Build history of the part. All positions in model axes, mm. Face numbers are marked on the shaded views. A direction names the side the tool comes from. Give positions to 0.01 mm unless a question says otherwise; leave off trailing zeros. Order: outer loops, then holes, each group sorted by start corner. A loop starts at its lowest first (then second) coordinate and runs counter-clockwise, first axis right, second up. Notation, with made-up numbers: (29.5, 72) - (45.5, 72) arc R29 cw to (45.5, 100) - close; hole circle Ø2 at (23, -2.5). An arc over 180 degrees is marked (long way). Use a Markdown table: item, result.
from build123d import *

# Parameters (mm, degrees)
SKETCH2_R          = 5.08
CUT_EXTRUDE1_DEPTH = 4.445
CUT_EXTRUDE2_DEPTH = 3.175
CIRPATTERN1_COUNT  = 5
CIRPATTERN1_ANGLE  = 300


with BuildPart() as part:
    # Sketch1 → Revolve1 (revolve)
    with BuildSketch(Plane.XY, mode=Mode.PRIVATE) as revolve1_sk:
        with BuildLine():
            Line((0, 0), (12.7, 0))
            Line((12.7, 0), (12.7, 3.175))
            Line((12.7, 3.175), (11.938, 3.175))
            ThreePointArc((11.938, 3.175), (11.324664102, 7.361873807), (10.16, 11.43))
            ThreePointArc((10.16, 11.43), (11.43, 12.7), (10.16, 13.97))
            ThreePointArc((10.16, 13.97), (7.163161242, 28.432586249), (6.35, 43.18))
            ThreePointArc((6.35, 43.18), (7.862457045, 46.853612737), (7.405308906, 50.8))
            Line((7.405308906, 50.8), (0, 50.8))
            Line((0, 50.8), (0, 0))
        make_face()
    revolve(revolve1_sk.sketch.rotate(Axis((0, 0, 0), (0, 1, 0)), 90), axis=Axis((0, 0, 0), (0, 1, 0)))

    # Sketch2 → Cut-Extrude1 (cut)
    with BuildSketch(Plane(origin=(0, 50.8, 0), x_dir=(1, 0, 0), z_dir=(0, 1, 0))):
        with Locations(Location((0, 0, 0), (0, 0, 270))):
            Circle(SKETCH2_R)
    extrude(amount=-CUT_EXTRUDE1_DEPTH, mode=Mode.SUBTRACT)

    # Sketch3 → Cut-Extrude2 (cut)
    with BuildSketch(Plane(origin=(0, 50.8, 0), x_dir=(1, 0, 0), z_dir=(0, 1, 0))):
        with BuildLine():
            Line((0, 10.16), (0, 5.08))
            ThreePointArc((0, 5.08), (-1.354819608, 4.896004885), (-2.611497409, 4.357347965))
            Line((-2.611497409, 4.357347965), (-5.070044486, 8.615676415))
            ThreePointArc((-5.070044486, 8.615676415), (-2.637496551, 9.724263362), (0, 10.16))
        make_face()
    cut_extrude2 = extrude(amount=-CUT_EXTRUDE2_DEPTH, mode=Mode.SUBTRACT)

    # CirPattern1: Cut-Extrude2 ×5 about axis
    cirpattern1_axis = Axis((0, 0, 0), (0, 1, 0))
    for i in range(1, CIRPATTERN1_COUNT):
        add(cut_extrude2.rotate(cirpattern1_axis, i * CIRPATTERN1_ANGLE / (CIRPATTERN1_COUNT - 1)), mode=Mode.SUBTRACT)


solid = part.part
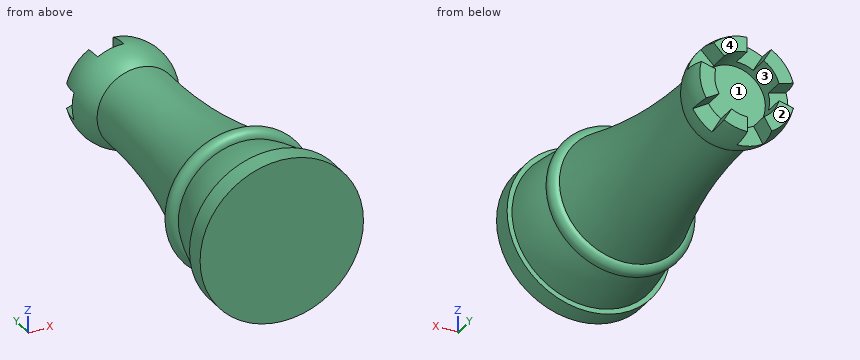
1) Slice it at B-B (y = 22.5). Write the cut outline in (x, z).
Computed:
| item | result |
|---|---|
| outline | circle Ø16.24 at (0, 0) |
2) Tool access for the marked faces 1 and 2: list every direction of +Z, -Z, +X, -X, +Y, -Y with a clear straight run to the whole face (end or side of a thin tool).
Computed:
| item | result |
|---|---|
| face 1 | +Y |
| face 2 | +Z, -Z, +X, -X, +Y |
3) Two-plate mould, pull along Z, no slides. Class the marked faces 3 and 4: +Z half, -Z half, draft (parallel to the pull), parting line (faces both ways), or undercut.
Computed:
| item | result |
|---|---|
| face 3 | undercut |
| face 4 | draft |
4) Pin check, flat tips, straight feed: P1, Ø0.9, axis at x = -6.5, z = 0.5, coming from the +Y side (3 decimals); P2, Ø8, axis at x = 0, z = 0, coming from the -Y side; P3, Ø3, axis at x = 6.5, y = 19, coming from the -Z side; P4, Ø0.9, axis at y = 48.5, z = 7, coming from the -X side. Stop position of each tip, or through.
Computed:
| item | result |
|---|---|
| P1 | stops at y = 47.625 |
| P2 | stops at y = 0 |
| P3 | stops at z = -7.4 |
| P4 | stops at x = -4.45 |
5) Slice it at A-A (y = 28.5). Write the cut outline in (x, z), and give its area (3 significant figures).
Computed:
| item | result |
|---|---|
| outline | circle Ø14.31 at (0, 0) |
| area | 161 mm² |
6) Wall check: line 1 (Y direction, x = -3.5, z = -2.5) (3 decimals); line 2 (X direction, y = 48, z = 0); line 3 (X direction, y = 46.5, z = 0.5). Give the ranges that are in metal, low to high. Write a range as from..to.
Computed:
| item | result |
|---|---|
| line 1 | y = 0..46.355 |
| line 2 | x = 5.08..7.94 |
| line 3 | x = -7.79..-5.06, 5.06..7.79 |
